Design review of the part built by this model. Coordinates are the model's own, in mm. Face numbers are marked on the shaded views. A direction names the side the tool comes from. Round coordinates to 2 decimals unless told otherwise and drop trailing zeros. Write each loop counter-clockwise with the first axis right and the second up, starting at its lowest first coordinate (ties: lowest second). Pieces come first, ordered by that corner, then holes. Notation, with made-up numbers: M 79.5,10.5 L 138.5,10.5 A22 ccw 138.5,47.5 Z; hole C -24.5,-39 d10. An arc over 180 degrees is marked long. Use CSV: the item, a comma, the result in double quotes.
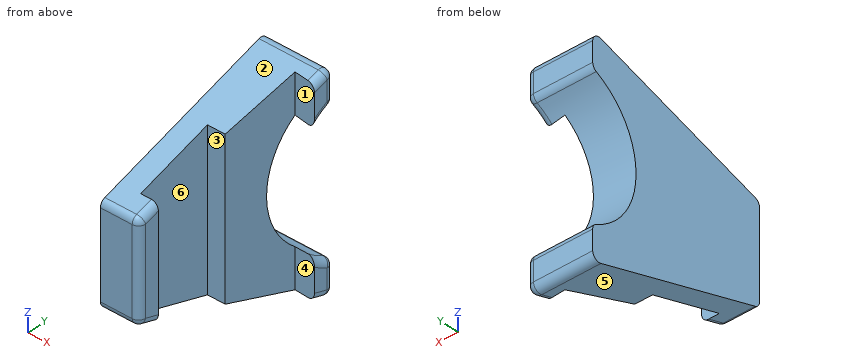
from build123d import *

# Parameters (mm, degrees)
F1_DEPTH = 15
F3_DEPTH = 9.3644707295
F4_R     = 1
F5_R     = 1


with BuildPart() as f1:
    # F0 (on Top) → F1 (new body, symmetric)
    with BuildSketch(Plane.XY):
        Polygon((0, 1.8765421212), (0.8748866353, 11.8765421212), (3.8634707295, 11.6150748929), (3.8634707295, 14.6150748929), (-5.5, 14.6150748929), (-5.5, -11.6234578788), (0, -11.6234578788), (0, -8.6234578788), (-2.5, -8.6234578788), (-2.5, 1.8765421212), align=None)
    extrude(amount=F1_DEPTH, both=True)

    # F2 (on face) → F3 (cut, through all)
    with BuildSketch(Plane(origin=(-5.5, 0, 0), x_dir=(0, -1, 0), z_dir=(-1, 0, 0))):
        Polygon((11.6234578788, -15), (11.6234578788, -6.8473624997), (-14.6150748929, -15), align=None)
        Polygon((11.6234578788, 15), (-14.6150748929, 15), (11.6234578788, 6.8473624997), align=None)
        with BuildLine():
            ThreePointArc((-14.6150748929, -10.1750748602), (-7.8033444248, 0), (-14.6150748929, 10.1750748602))
            Line((-14.6150748929, 10.1750748602), (-14.6150748929, -10.1750748602))
        make_face()
    extrude(amount=-F3_DEPTH, mode=Mode.SUBTRACT)

    # F4
    f4_edges = [f1.edges().sort_by_distance(p)[0] for p in [
        (-0.818265, 14.615075, 15),
        (-0.818265, 14.615075, -10.175075),
        (-0.818265, 14.615075, 10.175075),
        (-0.818265, 14.615075, -15),
        (-2.75, -11.623458, -6.847362),
        (-2.75, -11.623458, 6.847362),
    ]]
    fillet(f4_edges, radius=F4_R)

    # F5
    f5_edges = [f1.edges().sort_by_distance(p)[0] for p in [
        (3.863471, 14.615075, -12.232986),
        (3.863471, 14.615075, 12.232986),
        (0, -11.623458, 0),
    ]]
    fillet(f5_edges, radius=F5_R)


solid = f1.part
1) For pin 1 Ø5 at (x, y) = (-3, -7) entering from -Z; pin 2 Ø8 at (y, z) = (7.5, -2) entering from +X; pin 3 Ø8.5 at (y, z) = (-2.5, -4) entering from +X; pin 4 Ø3 at (x, z) = (2.5, 5.5) entering from -Y, all flat-tipped, find the tip position at first contact; note any pin that passes through.
Answers:
pin 1,"z = -9.06"
pin 2,"x = 0.65"
pin 3,"x = -2.5"
pin 4,"through"
2) Add section B-B on y = 10.75. Write out the cut boundary in (x, z).
Answers:
outline,"M -5.5,-13.8 L 0.78,-13.8 L 0.78,-7.5 L -5.5,-7.5 Z; M -5.5,7.5 L 0.78,7.5 L 0.78,13.8 L -5.5,13.8 Z"
3) The part is to be moulded in two halves that separate along X. For the marked faces 4, 5 and 6, say which applies: released by +X, released by -X, zero draft, split by the parting line, or undercut.
Answers:
face 4,"undercut"
face 5,"zero draft"
face 6,"released by +X"
4) Add section D-D on x = 2.5. Write out the cut boundary in (y, z).
Answers:
outline,"M 11.73,-14.1 L 13.32,-14.6 A1 ccw 14.62,-13.64 L 14.62,-10.82 A1 ccw 14.05,-9.92 A11.01 cw 11.73,-8.43 Z; M 11.73,8.43 A11.01 cw 14.05,9.92 A1 ccw 14.62,10.82 L 14.62,13.64 A1 ccw 13.32,14.6 L 11.73,14.1 Z"
5) Add section C-C on z = -5.75. Write out the cut boundary in (x, y), then the cut area to 3 significant figures.
Answers:
outline,"M -5.5,-11.62 L -1,-11.62 A1 ccw 0,-10.62 L 0,-8.62 L -2.5,-8.62 L -2.5,1.88 L 0,1.88 L 0.66,9.42 L -5.5,9.42 Z"
area,"91.8 mm²"
6) Wall thickness on line 1 along X through (y, z) = (1.25, -6.5); line 2 along Z through (x, y) = (-3, 13.75); line 3 along Y through (x, z) = (-2, -4.5): over which ranges is each line inside the solid? List them lowest first. Write a range as [from, to].
Answers:
line 1,"[-5.5, -2.5]"
line 2,"[-14.63, -9.77], [9.77, 14.63]"
line 3,"[-11.62, -8.62], [1.88, 8.77]"
7) Machinability: for the marked faces 1, 2 and 3, which of the approach directions +Z, -Z, +X, -X, +Y, -Y give a long, thin tool a straight path to every point of the face, cutting with its end or side? Answer none if there is none.
Answers:
face 1,"+Z, -Z, -Y"
face 2,"+Z, +X, -X, -Y"
face 3,"+Z, -Z, +X"
8) Add section A-A on x = -2. Write out the cut boundary in (y, z), then the cut area to 3 significant figures.
Answers:
outline,"M -11.62,-6.11 A1 ccw -10.92,-7.07 L -8.62,-7.78 L -8.62,7.78 L -10.92,7.07 A1 ccw -11.62,6.11 Z; M 1.88,-11.04 L 13.32,-14.6 A1 ccw 14.62,-13.64 L 14.62,-10.82 A1 ccw 14.05,-9.92 A11.01 cw 14.05,9.92 A1 ccw 14.62,10.82 L 14.62,13.64 A1 ccw 13.32,14.6 L 1.88,11.04 Z"
area,"274 mm²"
